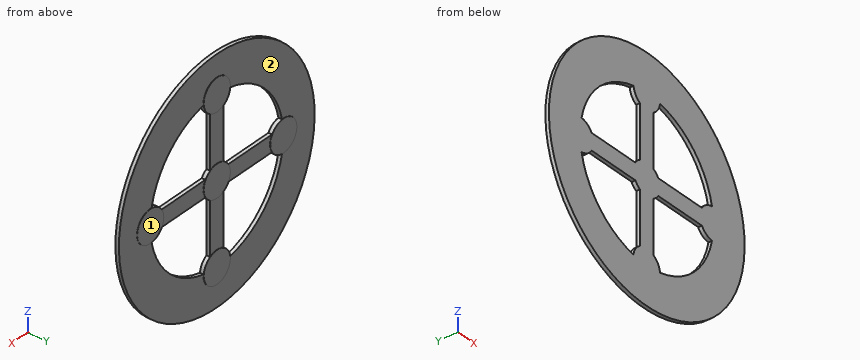
```python
from build123d import *

# Parameters (mm, degrees)
SKETCH2_R           = 550
BOSS_EXTRUDE1_DEPTH = 15
SKETCH3_OUTSIDE_W   = 1413.142
SKETCH3_OUTSIDE_H   = 1413.142
SKETCH3_OUTSIDE_R   = 500
CUT_EXTRUDE1_DEPTH  = 30
BOSS_EXTRUDE2_START = 1
SKETCH4_R           = 68
BOSS_EXTRUDE2_DEPTH = 1
CIRPATTERN1_COUNT   = 4
BOSS_EXTRUDE3_START = 1
SKETCH5_R           = 68
BOSS_EXTRUDE3_DEPTH = 1


with BuildPart() as part:
    # Sketch2 → Boss-Extrude1 (new body)
    with BuildSketch(Plane(origin=(0, 0, 0), x_dir=(1, 0, 0), z_dir=(0, 1, 0))):
        with Locations(Location((0, 0, 0), (0, 0, 270))):
            Circle(SKETCH2_R)
    extrude(amount=BOSS_EXTRUDE1_DEPTH)

    # Sketch3 outside → Cut-Extrude1 (cut)
    # profile 1 of 5: a face of its own
    with BuildSketch(Plane(origin=(0, 15, 0), x_dir=(1, 0, 0), z_dir=(0, 1, 0))):
        Rectangle(SKETCH3_OUTSIDE_W, SKETCH3_OUTSIDE_H)
        with Locations(Location((0, 0, 0), (0, 0, 270))):
            Circle(SKETCH3_OUTSIDE_R, mode=Mode.SUBTRACT)
    # profile 2 of 5: a face of its own
    with BuildSketch(Plane(origin=(0, 15, 0), x_dir=(1, 0, 0), z_dir=(0, 1, 0))):
        with BuildLine():
            Line((-35, 58.300943389), (-35, 281.699056611))
            ThreePointArc((-35, 281.699056611), (-57.426577842, 303.583133614), (-67.659145723, 333.2))
            ThreePointArc((-67.659145723, 333.2), (-240.416305603, 240.416305603), (-333.2, 67.659145723))
            ThreePointArc((-333.2, 67.659145723), (-303.583133614, 57.426577842), (-281.699056611, 35))
            Line((-281.699056611, 35), (-58.300943389, 35))
            ThreePointArc((-58.300943389, 35), (-48.083261121, 48.083261121), (-35, 58.300943389))
        make_face()
    # profile 3 of 5: a face of its own
    with BuildSketch(Plane(origin=(0, 15, 0), x_dir=(1, 0, 0), z_dir=(0, 1, 0))):
        with BuildLine():
            Line((35, 281.699056611), (35, 58.300943389))
            ThreePointArc((35, 58.300943389), (48.083261121, 48.083261121), (58.300943389, 35))
            Line((58.300943389, 35), (281.699056611, 35))
            ThreePointArc((281.699056611, 35), (303.583133614, 57.426577842), (333.2, 67.659145723))
            ThreePointArc((333.2, 67.659145723), (240.416305603, 240.416305603), (67.659145723, 333.2))
            ThreePointArc((67.659145723, 333.2), (57.426577842, 303.583133614), (35, 281.699056611))
        make_face()
    # profile 4 of 5: a face of its own
    with BuildSketch(Plane(origin=(0, 15, 0), x_dir=(1, 0, 0), z_dir=(0, 1, 0))):
        with BuildLine():
            Line((281.699056611, -35), (58.300943389, -35))
            ThreePointArc((58.300943389, -35), (48.083261121, -48.083261121), (35, -58.300943389))
            Line((35, -58.300943389), (35, -281.699056611))
            ThreePointArc((35, -281.699056611), (57.426577842, -303.583133614), (67.659145723, -333.2))
            ThreePointArc((67.659145723, -333.2), (240.416305603, -240.416305603), (333.2, -67.659145723))
            ThreePointArc((333.2, -67.659145723), (303.583133614, -57.426577842), (281.699056611, -35))
        make_face()
    # profile 5 of 5: a face of its own
    with BuildSketch(Plane(origin=(0, 15, 0), x_dir=(1, 0, 0), z_dir=(0, 1, 0))):
        with BuildLine():
            Line((-35, -281.699056611), (-35, -58.300943389))
            ThreePointArc((-35, -58.300943389), (-48.083261121, -48.083261121), (-58.300943389, -35))
            Line((-58.300943389, -35), (-281.699056611, -35))
            ThreePointArc((-281.699056611, -35), (-303.583133614, -57.426577842), (-333.2, -67.659145723))
            ThreePointArc((-333.2, -67.659145723), (-240.416305603, -240.416305603), (-67.659145723, -333.2))
            ThreePointArc((-67.659145723, -333.2), (-57.426577842, -303.583133614), (-35, -281.699056611))
        make_face()
    extrude(amount=-CUT_EXTRUDE1_DEPTH, mode=Mode.SUBTRACT)

    # Sketch4 → Boss-Extrude2 (add)
    with BuildSketch(Plane(origin=(0, 15, 0), x_dir=(1, 0, 0), z_dir=(0, 1, 0)).offset(BOSS_EXTRUDE2_START)):
        with Locations(Location((0, 340, 0), (0, 0, 270))):
            Circle(SKETCH4_R)
    boss_extrude2 = extrude(amount=-BOSS_EXTRUDE2_DEPTH)

    # CirPattern1: Boss-Extrude2 ×4 about axis
    cirpattern1_axis = Axis((0, 15, 0), (0, 1, 0))
    for i in range(1, CIRPATTERN1_COUNT):
        add(boss_extrude2.rotate(cirpattern1_axis, i * 360 / CIRPATTERN1_COUNT))

    # Sketch5 → Boss-Extrude3 (add)
    with BuildSketch(Plane(origin=(0, 15, 0), x_dir=(1, 0, 0), z_dir=(0, 1, 0)).offset(BOSS_EXTRUDE3_START)):
        with Locations(Location((0, 0, 0), (0, 0, 270))):
            Circle(SKETCH5_R)
    extrude(amount=-BOSS_EXTRUDE3_DEPTH)


solid = part.part
```
Model file for the job. Use its own axes, mm. Face numbers are marked on the shaded views. A direction names the side the tool comes from. Coordinates: 2 decimals unless noted, no trailing zeros. Loops run counter-clockwise (first coordinate to the right, second up) from the corner with the lowest first, then second, coordinate; pieces in that order, holes last. Notation, with made-up numbers: (77.25, 63) - (94.25, 63) arc R31 cw to (94.25, 100) - close; hole circle Ø5 at (65.5, 63.25). An arc over 180 degrees is marked (long way). Answer as a JSON object with one key per item and string values. Group by question number.
(1) Tool access for the marked faces 1 and 2: list every direction of +Z, -Z, +X, -X, +Y, -Y with a clear straight run to the whole face (end or side of a thin tool).
(2) Probe line 1 along Z through (x, y) = (179.5, 4.5); line 2 along X through (y, z) = (8.5, -62.5); line 3 along X through (y, z) = (5.25, 220.5). List the from-to ranges inside material, lowest first.
(3) Cut at A-A (y = 10). Give the cut face in (x, z), then the cut area to 3 significant figures.
(4) Cut at B-B (x = -258.5). Give the cut face in (y, z).
(5) Flat gauge pins, fed straight in: pin 1 (4.5 mm diameter, centred on y = 5, z = -152, fed in from +X); pin 2 (5 mm diameter, centred on x = 274.5, y = 9, fed in from +Z); pin 3 (6 mm diameter, centred on x = 48.5, y = 5, fed in from +Z). Where does each tip first touch, or does it go through?
(6) Cut at D-D (z = 0). Give the cut face in (x, y).
(7) Cut at C-C (z = 150.5). Give the cut face in (x, y).
Geometry says:
{
 "1": {"face 1": "+Z, -Z, +X, -X, +Y", "face 2": "+Y"},
 "2": {"line 1": "z = -466.67 to -288.76, -35 to 35, 288.76 to 466.67", "line 2": "x = -496.08 to -313.21, -35 to 35, 313.21 to 496.08", "line 3": "x = -448.75 to -258.8, -35 to 35, 258.8 to 448.75"},
 "3": {"outline": "circle Ø1000 at (0, 0); hole (-333.2, -67.66) arc R340 ccw to (-67.66, -333.2) arc R68 cw to (-35, -281.7) - (-35, -58.3) arc R68 cw to (-58.3, -35) - (-281.7, -35) arc R68 cw to start; hole (-333.2, 67.66) arc R68 cw to (-281.7, 35) - (-58.3, 35) arc R68 cw to (-35, 58.3) - (-35, 281.7) arc R68 cw to (-67.66, 333.2) arc R340 ccw to start; hole (35, -281.7) arc R68 cw to (67.66, -333.2) arc R340 ccw to (333.2, -67.66) arc R68 cw to (281.7, -35) - (58.3, -35) arc R68 cw to (35, -58.3) - close; hole (35, 58.3) arc R68 cw to (58.3, 35) - (281.7, 35) arc R68 cw to (333.2, 67.66) arc R340 ccw to (67.66, 333.2) arc R68 cw to (35, 281.7) - close", "area": "523,000 mm^2"},
 "4": {"outline": "(0, -427.99) - (15, -427.99) - (15, -220.86) - (0, -220.86) - close; (0, -35) - (15, -35) - (15, 35) - (0, 35) - close; (0, 220.86) - (15, 220.86) - (15, 427.99) - (0, 427.99) - close"},
 "5": {"pin 1": "stops at x = 477.05", "pin 2": "stops at z = 419.54", "pin 3": "stops at z = 497.93"},
 "6": {"outline": "(-500, 0) - (500, 0) - (500, 15) - (408, 15) - (408, 16) - (272, 16) - (272, 15) - (68, 15) - (68, 16) - (-68, 16) - (-68, 15) - (-272, 15) - (-272, 16) - (-408, 16) - (-408, 15) - (-500, 15) - close"},
 "7": {"outline": "(-476.81, 0) - (-304.88, 0) - (-304.88, 15) - (-476.81, 15) - close; (-35, 0) - (35, 0) - (35, 15) - (-35, 15) - close; (304.88, 0) - (476.81, 0) - (476.81, 15) - (304.88, 15) - close"}
}
